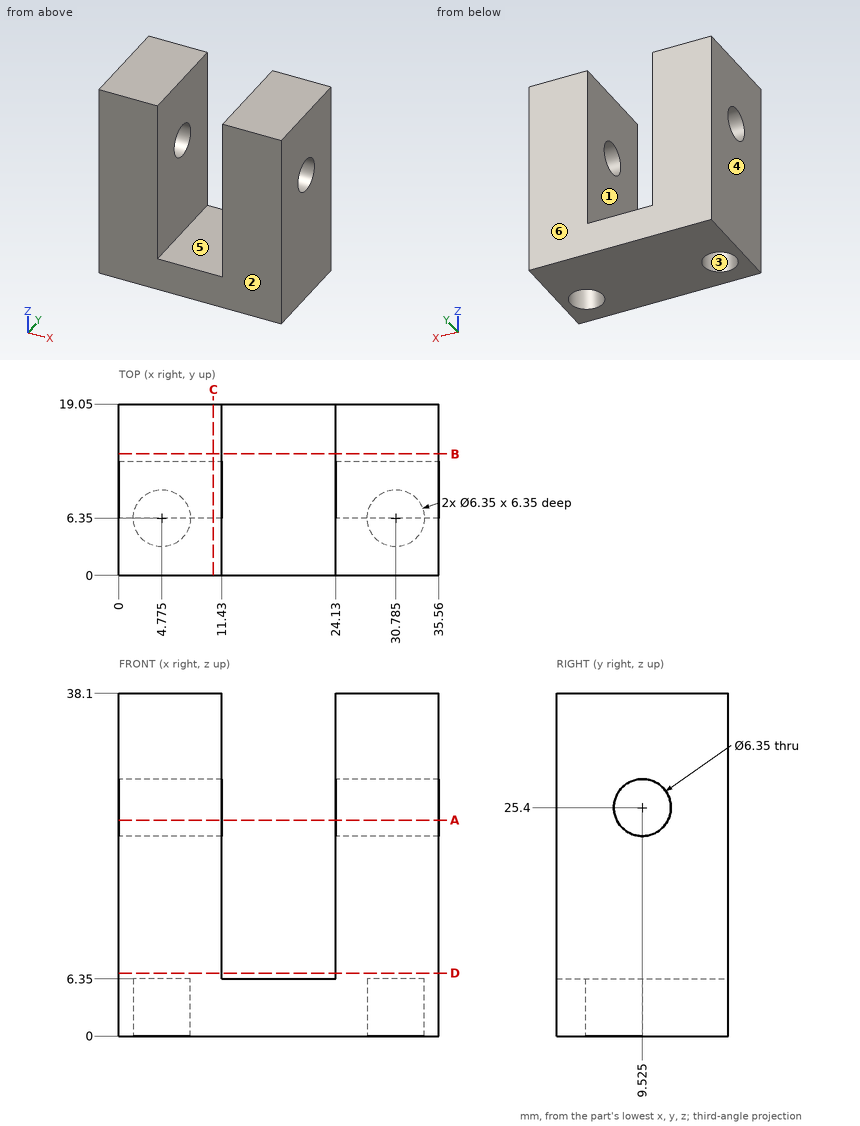
Design review of the part shown in the three views and the two pictorial views. Dimensions are in mm from the part's minimum x, y and z. A direction names the side the tool comes from. Round coordinates to 2 decimals unless told otherwise and drop trailing zeros. Loops run counter-clockwise (first coordinate to the right, second up) from the corner with the lowest first, then second, coordinate; pieces in that order, holes last. Notation, with made-up numbers: (82.25, 23) -> (127.25, 23) arc R11 cw to (127.25, 38) -> close; hole circle Ø1 at (39, 74). An arc over 180 degrees is marked (long way). Use one line per item in the form item = value. Start each with the question number.
Q1. Draft analysis for pull direction X (two halves, no side actions). For the marked faces 4, 5 and 6, state which applies: +X half, -X half, draft (parallel to the pull), parting line (faces both ways), or undercut.
Q2. For pin 1 Ø5 at (y, z) = (9.525, 25.4) entering from -X; pin 2 Ø1 at (x, y) = (20, 2) entering from +Z; pin 3 Ø3 at (x, y) = (29.5, 6) entering from -Z, all flat-tipped, find the tip position at first contact; note any pin that passes through.
Q3. We need section A-A on z = 24. State how many separate pieces and enclosed holes the cut face has, then the cut area to 3 significant figures.
Q4. Wall thickness on line 1 along X through (y, z) = (6, 34); line 2 along Y through (x, z) = (7.75, 25.4); line 3 along Y through (x, z) = (27.5, 28): over which ranges is each line inside the solid? List them lowest first. Write a range as [from, to].
Q5. We need section D-D on z = 7. Give the boundary of the cut face in (x, y).
Q6. We need section C-C on x = 10.5. Give the boundary of the cut face in (y, z) (3 decimals), then the cut area to 3 significant figures.
Q7. We need section B-B on y = 13.5. Give the boundary of the cut face in (x, z), then the cut area to 3 significant figures.
Q8. Machinability: for the marked faces 1, 2 and 3, which of the approach directions +Z, -Z, +X, -X, +Y, -Y give a long, thin tool a straight path to every point of the face, cutting with its end or side? Answer none if there is none.
Calculated:
q1.face_4 = -X half
q1.face_5 = undercut
q1.face_6 = draft
q2.pin_1 = through
q2.pin_2 = 6.35
q2.pin_3 = 6.35
q3.separate_pieces = 4
q3.enclosed_holes = 0
q3.area = 305 mm²
q4.line_1 = [0, 11.43], [24.13, 35.56]
q4.line_2 = [0, 6.35], [12.7, 19.05]
q4.line_3 = [0, 7.7], [11.35, 19.05]
q5.outline = (0, 0) -> (11.43, 0) -> (11.43, 19.05) -> (0, 19.05) -> close; (24.13, 0) -> (35.56, 0) -> (35.56, 19.05) -> (24.13, 19.05) -> close
q6.outline = (0, 0) -> (19.05, 0) -> (19.05, 38.1) -> (0, 38.1) -> close; hole circle Ø6.35 at (9.525, 25.4)
q6.area = 694 mm²
q7.outline = (0, 0) -> (35.56, 0) -> (35.56, 38.1) -> (24.13, 38.1) -> (24.13, 6.35) -> (11.43, 6.35) -> (11.43, 38.1) -> (0, 38.1) -> close
q7.area = 952 mm²
q8.face_1 = +Z, +Y, -Y
q8.face_2 = +Z, -Z, +X, -X, -Y
q8.face_3 = -Z
